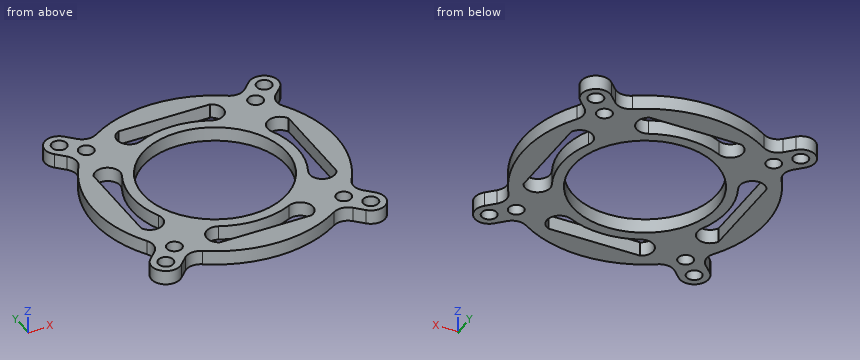
from build123d import *

# Parameters (mm, degrees)
SKETCH_1_R      = 2.1
SKETCH_1_R_2    = 20
EXTRUDE_1_DEPTH = 4


with BuildPart() as part:
    # 草图1 → 凸台-拉伸1 (new body)
    with BuildSketch(Plane.XY):
        with BuildLine():
            Line((49.221320344, -54.878174593), (46.870064467, -52.526918716))
            ThreePointArc((46.870064467, -52.526918716), (44.466937039, -51.378020085), (41.875216056, -51.992814233))
            ThreePointArc((41.875216056, -51.992814233), (23.55, -57.385), (5.224783944, -51.992814233))
            ThreePointArc((5.224783944, -51.992814233), (2.633062961, -51.378020085), (0.229935533, -52.526918716))
            Line((0.229935533, -52.526918716), (-2.121320344, -54.878174593))
            ThreePointArc((-2.121320344, -54.878174593), (-7.778174593, -54.878174593), (-7.778174593, -49.221320343))
            Line((-7.778174593, -49.221320343), (-5.426918716, -46.870064467))
            ThreePointArc((-5.426918716, -46.870064467), (-4.278020085, -44.466937039), (-4.892814234, -41.875216055))
            ThreePointArc((-4.892814234, -41.875216055), (-10.285, -23.55), (-4.892814233, -5.224783944))
            ThreePointArc((-4.892814233, -5.224783944), (-4.278020085, -2.633062961), (-5.426918716, -0.229935533))
            Line((-5.426918716, -0.229935533), (-7.778174593, 2.121320344))
            ThreePointArc((-7.778174593, 2.121320344), (-7.778174593, 7.778174593), (-2.121320343, 7.778174593))
            Line((-2.121320343, 7.778174593), (0.229935534, 5.426918716))
            ThreePointArc((0.229935534, 5.426918716), (2.633062961, 4.278020085), (5.224783945, 4.892814234))
            ThreePointArc((5.224783945, 4.892814234), (23.55, 10.285), (41.875216056, 4.892814233))
            ThreePointArc((41.875216056, 4.892814233), (44.466937039, 4.278020085), (46.870064467, 5.426918716))
            Line((46.870064467, 5.426918716), (49.221320344, 7.778174593))
            ThreePointArc((49.221320344, 7.778174593), (54.878174593, 7.778174593), (54.878174593, 2.121320344))
            Line((54.878174593, 2.121320344), (52.526918716, -0.229935533))
            ThreePointArc((52.526918716, -0.229935533), (51.378020085, -2.633062961), (51.992814234, -5.224783945))
            ThreePointArc((51.992814234, -5.224783945), (57.385, -23.55), (51.992814233, -41.875216056))
            ThreePointArc((51.992814233, -41.875216056), (51.378020085, -44.466937039), (52.526918716, -46.870064467))
            Line((52.526918716, -46.870064467), (54.878174593, -49.221320344))
            ThreePointArc((54.878174593, -49.221320344), (54.878174593, -54.878174593), (49.221320344, -54.878174593))
        make_face()
        with Locations((47.1, -47.1)):
            Circle(SKETCH_1_R, mode=Mode.SUBTRACT)
        with Locations((23.55, -23.55)):
            Circle(SKETCH_1_R_2, mode=Mode.SUBTRACT)
        with Locations((52.049747468, -52.049747468)):
            Circle(SKETCH_1_R, mode=Mode.SUBTRACT)
        with Locations((-4.949747468, -52.049747468)):
            Circle(SKETCH_1_R, mode=Mode.SUBTRACT)
        with Locations((-4.949747468, 4.949747468)):
            Circle(SKETCH_1_R, mode=Mode.SUBTRACT)
        with Locations((52.049747468, 4.949747468)):
            Circle(SKETCH_1_R, mode=Mode.SUBTRACT)
        with Locations((0, -47.1)):
            Circle(SKETCH_1_R, mode=Mode.SUBTRACT)
        Circle(SKETCH_1_R, mode=Mode.SUBTRACT)
        with Locations((47.1, 0)):
            Circle(SKETCH_1_R, mode=Mode.SUBTRACT)
        with BuildLine():
            Line((10.774989316, 3.594043583), (36.325010684, 3.594043583))
            ThreePointArc((36.325010684, 3.594043583), (38.001397856, -1.063179415), (33.344174858, -2.739566587))
            ThreePointArc((33.344174858, -2.739566587), (23.55, -0.55), (13.755825142, -2.739566587))
            ThreePointArc((13.755825142, -2.739566587), (9.098602144, -1.063179415), (10.774989316, 3.594043583))
        make_face(mode=Mode.SUBTRACT)
        with BuildLine():
            Line((-3.594043583, -36.325010684), (-3.594043583, -10.774989316))
            ThreePointArc((-3.594043583, -10.774989316), (1.063179415, -9.098602144), (2.739566587, -13.755825142))
            ThreePointArc((2.739566587, -13.755825142), (0.55, -23.55), (2.739566587, -33.344174858))
            ThreePointArc((2.739566587, -33.344174858), (1.063179415, -38.001397856), (-3.594043583, -36.325010684))
        make_face(mode=Mode.SUBTRACT)
        with BuildLine():
            Line((10.774989316, -50.694043583), (36.325010684, -50.694043583))
            ThreePointArc((36.325010684, -50.694043583), (38.001397856, -46.036820585), (33.344174858, -44.360433413))
            ThreePointArc((33.344174858, -44.360433413), (23.55, -46.55), (13.755825142, -44.360433413))
            ThreePointArc((13.755825142, -44.360433413), (9.098602144, -46.036820585), (10.774989316, -50.694043583))
        make_face(mode=Mode.SUBTRACT)
        with BuildLine():
            Line((50.694043583, -10.774989316), (50.694043583, -36.325010684))
            ThreePointArc((50.694043583, -36.325010684), (46.036820585, -38.001397856), (44.360433413, -33.344174858))
            ThreePointArc((44.360433413, -33.344174858), (46.55, -23.55), (44.360433413, -13.755825142))
            ThreePointArc((44.360433413, -13.755825142), (46.036820585, -9.098602144), (50.694043583, -10.774989316))
        make_face(mode=Mode.SUBTRACT)
    extrude(amount=EXTRUDE_1_DEPTH)


solid = part.part
Work out the finished part from the listing and answer in its coordinate system (mm). Give positions to 0.01 mm unless a question says otherwise; leave off trailing zeros. Write each loop counter-clockwise with the first axis right and the second up, starting at its lowest first coordinate (ties: lowest second). Pieces come first, ordered by that corner, then holes.
Q1. The part is cut by section A-A on y = -23.55. Give the vertices of the cut face in (x, z) (3 decimals), and give its area (3 significant figures).
Answer:
outline: (-10.285, 0) - (-3.594, 0) - (-3.594, 4) - (-10.285, 4) - close; (0.55, 0) - (3.55, 0) - (3.55, 4) - (0.55, 4) - close; (43.55, 0) - (46.55, 0) - (46.55, 4) - (43.55, 4) - close; (50.694, 0) - (57.385, 0) - (57.385, 4) - (50.694, 4) - close
area: 77.5 mm2
Q2. Straight lines are drawn through the part: L1, parallel to Y at x = 24, z = 3.6; L2, parallel to Y at x = 27, z = 3.2; L3, parallel to X at y = -2.5, z = 2. For each, find the intervals that lie inside material, in ascending order.
Answer:
L1: y = -57.38 to -50.69, -46.55 to -43.54, -3.56 to -0.55, 3.59 to 10.28
L2: y = -57.21 to -50.69, -46.29 to -43.25, -3.85 to -0.81, 3.59 to 10.11
L3: x = -4.29 to 10.35, 14.28 to 32.82, 36.75 to 51.39
Q3. The part is cut by section B-B on x = 23.55. Give the vertices of the cut face in (y, z) (3 decimals), and give its area (3 significant figures).
Answer:
outline: (-57.385, 0) - (-50.694, 0) - (-50.694, 4) - (-57.385, 4) - close; (-46.55, 0) - (-43.55, 0) - (-43.55, 4) - (-46.55, 4) - close; (-3.55, 0) - (-0.55, 0) - (-0.55, 4) - (-3.55, 4) - close; (3.594, 0) - (10.285, 0) - (10.285, 4) - (3.594, 4) - close
area: 77.5 mm2
Q4. Given pin 1 (2.5 mm diameter, centred on x = 47.1, y = -47.1, fed in from -Z); pin 2 (1.2 mm diameter, centred on y = -25, z = 2, fed in from -X); pin 3 (2 mm diameter, centred on x = 29, z = 1.5, fed in from +Y); pin 4 (2 mm diameter, centred on x = 47.5, z = 2, fed in from -Y), each flat-ended and moving along its own axis, determine where each tip first touches the part or whether it passes through.
Answer:
pin 1: passes through
pin 2: stops at x = -10.27
pin 3: stops at y = 9.99
pin 4: stops at y = -54.16
Q5. The part is cut by section C-C on z = 1.6. State how many separate pieces and enclosed holes the cut face has, and give its area (3 significant figures).
Answer:
separate pieces: 1
enclosed holes: 13
area: 1,950 mm2
